Design review of the part shown in the three views and the two pictorial views. Dimensions are in mm from the part's minimum x, y and z. Coordinates: 2 decimals unless noted, no trailing zeros. Loops run counter-clockwise (first coordinate to the right, second up) from the corner with the lowest first, then second, coordinate; pieces in that order, holes last.
Q1. Add section D-D on z = 52. Give the boundary of the cut face in (x, y).
Q2. Add section B-B on x = 40. Give the boundary of the cut face in (y, z).
Q3. Add section C-C on y = 0.95. Give the boundary of the cut face in (x, z).
Q4. Add section A-A on z = 40. Give the boundary of the cut face in (x, y), and give its area (3 significant figures).
Q5. For P1, Ø1, axis at y = 1, z = 63, coming from the -X side; P2, Ø4, axis at x = 67.5, z = 46, coming from the -Y side; P3, Ø1.5, axis at x = 49, y = 1.5, coming from the -Z side, all flat-tipped, find the tip position at first contact; note any pin that passes through.
Q6. Wall thickness on probe 1 along Z at (x, y) = (40, 1.75); probe 2 along X at (y, z) = (0.2, 45.5); probe 3 along Z at (x, y) = (39, 2.55): over which ranges is each line inside the solid? List them lowest first.
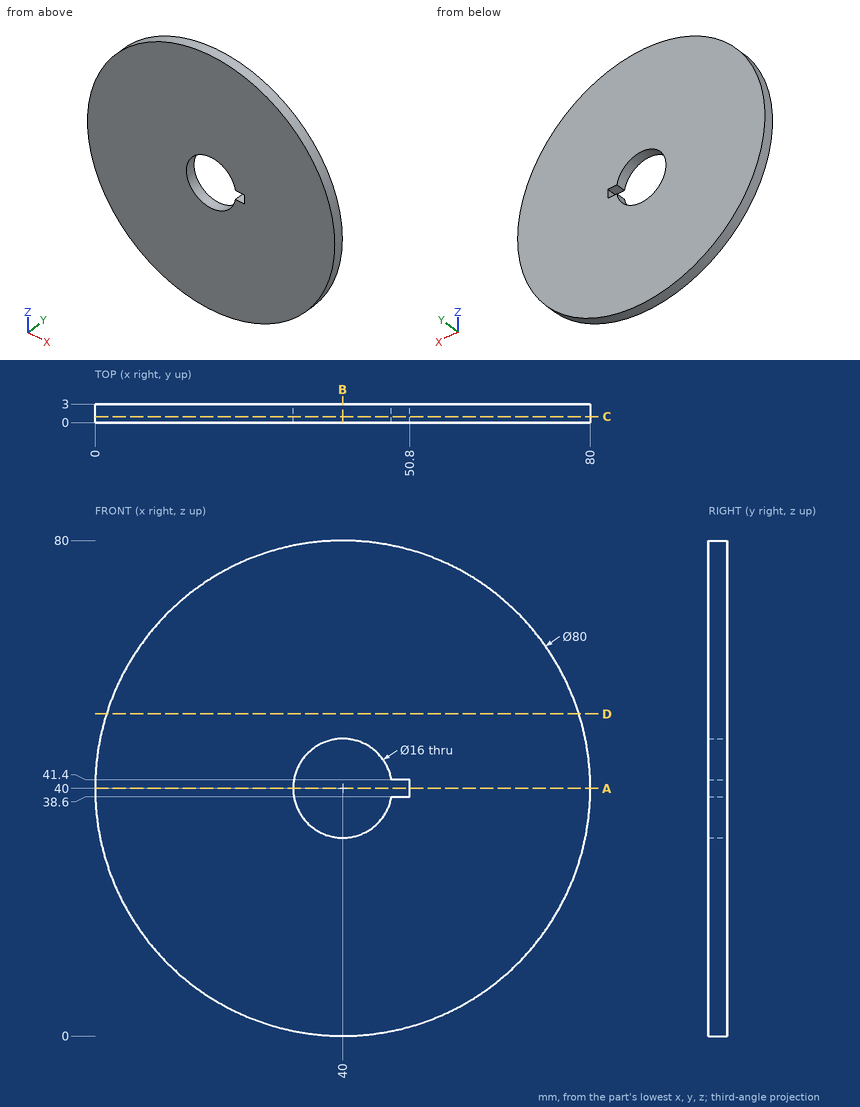
Entries:
1. outline: (1.84, 0) - (78.16, 0) - (78.16, 3) - (1.84, 3) - close
2. outline: (0, 0) - (3, 0) - (3, 32) - (0, 32) - close; (0, 48) - (3, 48) - (3, 80) - (0, 80) - close
3. outline: circle Ø80 at (40, 40); hole (47.88, 38.6) - (50.8, 38.6) - (50.8, 41.4) - (47.88, 41.4) arc R8 ccw (long way) to start
4. outline: (0, 0) - (32, 0) - (32, 3) - (0, 3) - close; (50.8, 0) - (80, 0) - (80, 3) - (50.8, 3) - close
4. area: 184 mm2
5. P1: stops at x = 6.93
5. P2: stops at y = 0
5. P3: stops at z = 0.86
6. probe 1: z = 0 to 32, 48 to 80
6. probe 2: x = 0.38 to 34.19, 45.81 to 79.62
6. probe 3: z = 0.01 to 32.06, 47.94 to 79.99
